The model under review builds one solid part; all positions refer to its coordinate system, in mm. A direction names the side the tool comes from. Round coordinates to 2 decimals unless told otherwise and drop trailing zeros. Write each loop counter-clockwise with the first axis right and the second up, starting at its lowest first coordinate (ties: lowest second). Pieces come first, ordered by that corner, then holes. Notation, with made-up numbers: (7.25, 45.5) - (56.25, 45.5) arc R12 ccw to (56.25, 55.5) - close; hole circle Ø2 at (-22.75, 35.5). An arc over 180 degrees is marked (long way). Return JSON: item names as keys, results as strings.
from build123d import *

# Parameters (mm, degrees)
BOSS_EXTRUDE1_DEPTH = 5
CUT_EXTRUDE2_DEPTH  = 2.5
CUT_EXTRUDE6_START  = -2.5
CUT_EXTRUDE6_DEPTH  = 2.5
SKETCH11_R          = 2.5
CUT_EXTRUDE7_DEPTH  = 2.5
SKETCH12_R          = 2.5
BOSS_EXTRUDE3_DEPTH = 2.5


# Read off the part's stored shape, not the designer's step: Cut-Extrude6
with BuildPart() as part:
    # Sketch1 → Boss-Extrude1 (new body)
    with BuildSketch(Plane.XY):
        with BuildLine():
            Line((0, 0), (20, 0))
            ThreePointArc((20, 0), (27.5, 7.5), (20, 15))
            Line((20, 15), (0, 15))
            ThreePointArc((0, 15), (-7.5, 7.5), (0, 0))
        make_face()
    extrude(amount=BOSS_EXTRUDE1_DEPTH)

    # Sketch6 → Cut-Extrude2 (cut)
    with BuildSketch(Plane(origin=(0, 0, 0), x_dir=(-1, 0, 0), z_dir=(0, 0, -1))):
        with BuildLine():
            Line((-20, 15), (-12.5, 15))
            Line((-12.5, 15), (-12.5, 0))
            Line((-12.5, 0), (-20, 0))
            ThreePointArc((-20, 0), (-27.5, 7.5), (-20, 15))
        make_face()
    extrude(amount=-CUT_EXTRUDE2_DEPTH, mode=Mode.SUBTRACT)

    # Cut-Extrude6 outline → Cut-Extrude6 (cut)
    with BuildSketch(Plane.XY.offset(5).offset(CUT_EXTRUDE6_START)):
        with BuildLine():
            Line((7.746832871, 0), (7.746832871, 15))
            Line((7.746832871, 15), (0, 15))
            ThreePointArc((0, 15), (-7.5, 7.5), (0, 0))
            Line((0, 0), (7.746832871, 0))
        make_face()
    extrude(amount=CUT_EXTRUDE6_DEPTH, mode=Mode.SUBTRACT)

    # Sketch11 → Cut-Extrude7 (cut)
    with BuildSketch(Plane.XY.offset(2.5)):
        with Locations((0, 7.5)):
            Circle(SKETCH11_R)
    extrude(amount=-CUT_EXTRUDE7_DEPTH, mode=Mode.SUBTRACT)

    # Sketch12 → Boss-Extrude3 (add)
    with BuildSketch(Plane(origin=(0, 0, 2.5), x_dir=(-1, 0, 0), z_dir=(0, 0, -1))):
        with Locations((-20, 7.5)):
            Circle(SKETCH12_R)
    extrude(amount=BOSS_EXTRUDE3_DEPTH)


solid = part.part
(1) Add section A-A (z = 1.75). Write out the cut boundary in (x, y), plus the area to 3 significant figures.
Filled in:
{"outline": "(0, 0) - (12.5, 0) - (12.5, 15) - (0, 15) arc R7.5 ccw to start; circle Ø5 at (20, 7.5); hole circle Ø5 at (0, 7.5)", "area": "276 mm2"}
(2) Clearance check with flat-ended pins moving along their axes: pin 1 Ø3 at (x, z) = (21, 2) entering from +Y; pin 2 Ø1.5 at (y, z) = (2.5, 4) entering from -X. State where each tip first meets the part, or that it passes through.
Filled in:
{"pin 1": "stops at y = 15", "pin 2": "stops at x = 7.75"}
(3) Add section D-D (x = 22). Write out the cut boundary in (y, z), plus the area to 3 significant figures.
Filled in:
{"outline": "(0.27, 2.5) - (6, 2.5) - (6, 0) - (9, 0) - (9, 2.5) - (14.73, 2.5) - (14.73, 5) - (0.27, 5) - close", "area": "43.6 mm2"}
(4) Wall thickness on line 1 (Y direction, x = 0, z = 1.4); line 2 (Z direction, x = 4, y = 1); line 3 (Z direction, x = 19, y = 1): over which ranges is each line inside the solid? List them lowest first.
Filled in:
{"line 1": "y = 0 to 5, 10 to 15", "line 2": "z = 0 to 2.5", "line 3": "z = 2.5 to 5"}
(5) For faces 1 (the flat face through (12.5, 8, 1)), 2 (the cylindrical face through (22, 6, 1)), 3 (the flat face through (7.747, 7, 4)), list the 3-axis set-ups (+Z, -Z, +X, -X, +Y, -Y) from which the entire face can be reached by the end or side of a thin tool; tool diameter is ignored.
Filled in:
{"face 1": "-Z, +Y, -Y", "face 2": "-Z", "face 3": "+Z, -X, +Y, -Y"}
(6) Mouldability with a two-part tool opening along X and no side actions: class faces 4 (the cylindrical face through (-0.54, 5.06, 1.27)), 5 (the cylindrical face through (27.5, 7.34, 3.73)), 6 (the flat face through (10, 15, 2)) as released by +X, released by -X, zero draft, split by the parting line, or undercut.
Filled in:
{"face 4": "undercut", "face 5": "released by +X", "face 6": "zero draft"}
(7) Add section B-B (y = 7.5). Write out the cut boundary in (x, z), plus the area to 3 significant figures.
Filled in:
{"outline": "(-7.5, 0) - (-2.5, 0) - (-2.5, 2.5) - (-7.5, 2.5) - close; (2.5, 0) - (12.5, 0) - (12.5, 2.5) - (17.5, 2.5) - (17.5, 0) - (22.5, 0) - (22.5, 2.5) - (27.5, 2.5) - (27.5, 5) - (7.75, 5) - (7.75, 2.5) - (2.5, 2.5) - close", "area": "99.4 mm2"}
(8) Add section C-C (y = 3). Write out the cut boundary in (x, z), plus the area to 3 significant figures.
Filled in:
{"outline": "(-6, 0) - (12.5, 0) - (12.5, 2.5) - (26, 2.5) - (26, 5) - (7.75, 5) - (7.75, 2.5) - (-6, 2.5) - close", "area": "91.9 mm2"}
